Check sheet for the modelled part. Datum: model origin and axes. Units: mm. A direction names the side the tool comes from. Coordinates: 2 decimals unless noted, no trailing zeros. Loops run counter-clockwise (first coordinate to the right, second up) from the corner with the lowest first, then second, coordinate; pieces in that order, holes last. Notation, with made-up numbers: M 83,-13 L 120,-13 A3 cw 120,-9 Z; hole C 16,-9 d1. An arc over 180 degrees is marked long. Answer as CSV lines item,"result". Start each with the question number.
from build123d import *

# Parameters (mm, degrees)
SKETCH1_W           = 95
SKETCH1_H           = 150
BOSS_EXTRUDE1_DEPTH = 3.5
SKETCH2_W           = 5.5
SKETCH2_H           = 10
SKETCH2_W_2         = 10
SKETCH2_H_2         = 5.5
BOSS_EXTRUDE2_DEPTH = 10
CUT_EXTRUDE1_DEPTH  = 3
CUT_EXTRUDE2_DEPTH  = 3
SKETCH6_R           = 1.55
CUT_EXTRUDE3_DEPTH  = 10.5
SKETCH7_R           = 1.55
CUT_EXTRUDE4_DEPTH  = 10.5
SKETCH8_W           = 95
SKETCH8_H           = 150
SKETCH8_W_2         = 87
SKETCH8_H_2         = 142
BOSS_EXTRUDE3_DEPTH = 50
SKETCH9_W           = 60
SKETCH9_H           = 15
CUT_EXTRUDE5_DEPTH  = 50
SKETCH10_R          = 8.5
CUT_EXTRUDE6_DEPTH  = 50


with BuildPart() as part:
    # Sketch1 → Boss-Extrude1 (new body)
    with BuildSketch(Plane(origin=(0, 0, 0), x_dir=(1, 0, 0), z_dir=(0, 1, 0))):
        Rectangle(SKETCH1_W, SKETCH1_H)
    extrude(amount=BOSS_EXTRUDE1_DEPTH)

    # Sketch2 → Boss-Extrude2 (add)
    with BuildSketch(Plane(origin=(0, 3.5, 0), x_dir=(1, 0, 0), z_dir=(0, 1, 0))):
        with Locations((-40.75, 50)):
            Rectangle(SKETCH2_W, SKETCH2_H)
        with Locations((22.5, 68.25)):
            Rectangle(SKETCH2_W_2, SKETCH2_H_2)
    boss_extrude2 = extrude(amount=BOSS_EXTRUDE2_DEPTH)

    # Sketch3 → Cut-Extrude1 (cut)
    with BuildSketch(Plane.XY.offset(-65.5)):
        Polygon((22.5, 5.324573519), (25.25, 6.91228676), (25.25, 10.08771324), (22.5, 11.675426481), (19.75, 10.08771324), (19.75, 6.91228676), align=None)
    cut_extrude1 = extrude(amount=-CUT_EXTRUDE1_DEPTH, mode=Mode.SUBTRACT)

    # Sketch4 → Cut-Extrude2 (cut)
    with BuildSketch(Plane(origin=(-38, 0, 0), x_dir=(0, 0, -1), z_dir=(1, 0, 0))):
        Polygon((49.928125047, 5.324573519), (52.678125047, 6.91228676), (52.678125047, 10.08771324), (49.928125047, 11.675426481), (47.178125047, 10.08771324), (47.178125047, 6.91228676), align=None)
    cut_extrude2 = extrude(amount=-CUT_EXTRUDE2_DEPTH, mode=Mode.SUBTRACT)

    # Sketch6 → Cut-Extrude3 (cut, through all)
    with BuildSketch(Plane(origin=(-38, 0, 0), x_dir=(0, 0, -1), z_dir=(1, 0, 0))):
        with Locations((50, 8.5)):
            Circle(SKETCH6_R)
    cut_extrude3 = extrude(amount=-CUT_EXTRUDE3_DEPTH, mode=Mode.SUBTRACT)

    # Sketch7 → Cut-Extrude4 (cut, through all)
    with BuildSketch(Plane.XY.offset(-65.5)):
        with Locations((22.5, 8.5)):
            Circle(SKETCH7_R)
    cut_extrude4 = extrude(amount=-CUT_EXTRUDE4_DEPTH, mode=Mode.SUBTRACT)

    # Sketch8 → Boss-Extrude3 (add)
    with BuildSketch(Plane.XZ):
        Rectangle(SKETCH8_W, SKETCH8_H)
        Rectangle(SKETCH8_W_2, SKETCH8_H_2, mode=Mode.SUBTRACT)
    extrude(amount=BOSS_EXTRUDE3_DEPTH)

    # Sketch9 → Cut-Extrude5 (cut)
    with BuildSketch(Plane.XZ):
        with Locations((-0.026887888, -55)):
            Rectangle(SKETCH9_W, SKETCH9_H)
    cut_extrude5 = extrude(amount=-CUT_EXTRUDE5_DEPTH, mode=Mode.SUBTRACT)

    # Sketch10 → Cut-Extrude6 (cut)
    with BuildSketch(Plane(origin=(47.5, 0, 0), x_dir=(0, 0, -1), z_dir=(1, 0, 0))):
        with Locations((50, -11.5)):
            Circle(SKETCH10_R)
        with Locations((24, -11.5)):
            Circle(SKETCH10_R)
    cut_extrude6 = extrude(amount=-CUT_EXTRUDE6_DEPTH, mode=Mode.SUBTRACT)

    # Mirror1: Boss-Extrude2, Cut-Extrude1, Cut-Extrude2, Cut-Extrude3, Cut-Extrude4, Cut-Extrude5, Cut-Extrude6 across plane
    add(boss_extrude2.mirror(Plane.XY))
    add(cut_extrude1.mirror(Plane.XY), mode=Mode.SUBTRACT)
    add(cut_extrude2.mirror(Plane.XY), mode=Mode.SUBTRACT)
    add(cut_extrude3.mirror(Plane.XY), mode=Mode.SUBTRACT)
    add(cut_extrude4.mirror(Plane.XY), mode=Mode.SUBTRACT)
    add(cut_extrude5.mirror(Plane.XY), mode=Mode.SUBTRACT)
    add(cut_extrude6.mirror(Plane.XY), mode=Mode.SUBTRACT)


solid = part.part
Item 1: Sectioned sample at D-D, the plane y = -43. Record the boundary of the cut face in (x, z).
Item 2: Material ranges on line 1 (Y direction, x = 45.45, z = 50); line 2 (Z direction, x = 29.5, y = -33); line 3 (X direction, y = -31.5, z = 49.5), recorded low to high. Write a range as from..to.
Item 3: Sectioned sample at B-B, the plane x = -6.5. Record the boundary of the cut face in (y, z).
Item 4: Set-up check for faces 1 (the face through (-41, 7, 49)), 2 (the face through (43.5, -25, -1)), 3 (the face through (21, 7, -68.5)): record each of +Z, -Z, +X, -X, +Y, -Y from which the full face is reachable in a straight line by a thin tool's end or side.
Item 5: Go/stop test with flat-tipped pins: pin 1 (15.5 mm diameter, centred on y = -11.5, z = 24, fed in from +X); pin 2 (3 mm diameter, centred on x = -40, y = 6, fed in from +Z); pin 3 (1.6 mm diameter, centred on x = 21.5, y = 8.5, fed in from -Z). Record where each tip stops, or that it passes through.
Item 6: Sectioned sample at A-A, the plane y = -11.5. Record the boundary of the cut face in (x, z).
Item 7: Release check for a two-part mould opening along Y. For faces 4 (the face through (-42.232, 8.966, -51.478)), 5 (the face through (20, 6, 65.5)) record: released by +Y, released by -Y, zero draft, split by the parting line, or undercut.
Item 8: Sectioned sample at C-C, the plane z = 24. Record the boundary of the cut face in (x, y).
Reply:
1,outline,"M -47.5,-75 L 47.5,-75 L 47.5,75 L -47.5,75 Z; hole M -43.5,-71 L 43.5,-71 L 43.5,71 L -43.5,71 Z"
2,line 1,"-50..-20, -3..3.5"
2,line 2,"-75..-71, 71..75"
2,line 3,"-47.5..-43.5, 43.5..47.5"
3,outline,"M -50,-75 L 3.5,-75 L 3.5,-62.5 L 0,-62.5 L 0,-71 L -50,-71 Z; M -50,71 L 0,71 L 0,62.5 L 3.5,62.5 L 3.5,75 L -50,75 Z; M 0,-47.5 L 3.5,-47.5 L 3.5,47.5 L 0,47.5 Z"
4,face 1,"+X"
4,face 2,"-Y"
4,face 3,"none"
5,pin 1,"x = -43.5"
5,pin 2,"z = 55"
5,pin 3,"z = -71"
6,outline,"M -47.5,-75 L 47.5,-75 L 47.5,-58.5 L 43.5,-58.5 L 43.5,-71 L -43.5,-71 L -43.5,71 L 43.5,71 L 43.5,58.5 L 47.5,58.5 L 47.5,75 L -47.5,75 Z; M 43.5,-41.5 L 47.5,-41.5 L 47.5,-32.5 L 43.5,-32.5 Z; M 43.5,-15.5 L 47.5,-15.5 L 47.5,15.5 L 43.5,15.5 Z; M 43.5,32.5 L 47.5,32.5 L 47.5,41.5 L 43.5,41.5 Z"
7,face 4,"undercut"
7,face 5,"zero draft"
8,outline,"M -47.5,-50 L -43.5,-50 L -43.5,0 L 43.5,0 L 43.5,-3 L 47.5,-3 L 47.5,3.5 L -47.5,3.5 Z; M 43.5,-50 L 47.5,-50 L 47.5,-20 L 43.5,-20 Z"
